Can you work these out from the model? Positions are in its coordinate system, mm. Face numbers are marked on the shaded views. A direction names the side the tool comes from. Coordinates: 2 decimals unless noted, no trailing zeros. Loops run counter-clockwise (first coordinate to the right, second up) from the corner with the lowest first, then second, coordinate; pieces in that order, holes last.
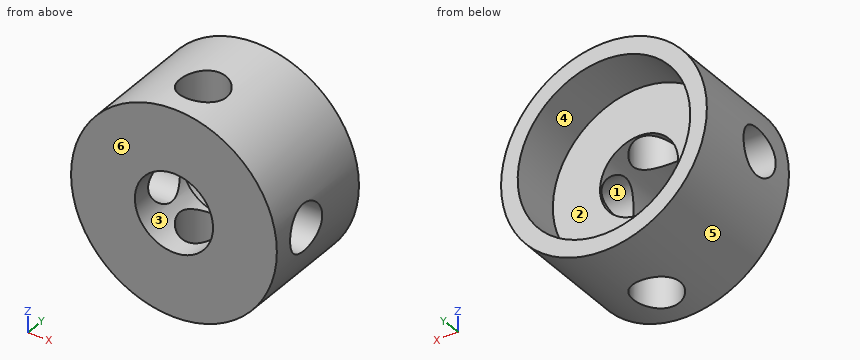
```python
from build123d import *

# Parameters (mm, degrees)
SKETCH1_R           = 7.62
SKETCH1_R_2         = 2.8956
BOSS_EXTRUDE1_DEPTH = 5.08
SKETCH2_R           = 7.62
SKETCH2_R_2         = 6.3881
BOSS_EXTRUDE2_DEPTH = 3.81
SKETCH3_R           = 1.7399
CUT_EXTRUDE1_DEPTH  = 12.7
SKETCH4_R           = 1.7399
CUT_EXTRUDE2_DEPTH  = 12.7


with BuildPart() as part:
    # Sketch1 → Boss-Extrude1 (new body)
    with BuildSketch(Plane(origin=(0, 0, 0), x_dir=(1, 0, 0), z_dir=(0, 1, 0))):
        with Locations(Location((0, 0, 0), (0, 0, 270))):
            Circle(SKETCH1_R)
        with Locations(Location((0, 0, 0), (0, 0, 270))):
            Circle(SKETCH1_R_2, mode=Mode.SUBTRACT)
    extrude(amount=BOSS_EXTRUDE1_DEPTH)

    # Sketch2 → Boss-Extrude2 (add)
    with BuildSketch(Plane(origin=(0, 5.08, 0), x_dir=(1, 0, 0), z_dir=(0, 1, 0))):
        with Locations(Location((0, 0, 0), (0, 0, 270))):
            Circle(SKETCH2_R)
        with Locations(Location((0, 0, 0), (0, 0, 90))):
            Circle(SKETCH2_R_2, mode=Mode.SUBTRACT)
    extrude(amount=BOSS_EXTRUDE2_DEPTH)

    # Sketch3 → Cut-Extrude1 (cut, symmetric)
    with BuildSketch(Plane.XY):
        with Locations((0, 3.175)):
            Circle(SKETCH3_R)
    extrude(amount=CUT_EXTRUDE1_DEPTH, both=True, mode=Mode.SUBTRACT)

    # Sketch4 → Cut-Extrude2 (cut, symmetric)
    with BuildSketch(Plane(origin=(0, 0, 0), x_dir=(0, 0, -1), z_dir=(1, 0, 0))):
        with Locations((0, 3.175)):
            Circle(SKETCH4_R)
    extrude(amount=CUT_EXTRUDE2_DEPTH, both=True, mode=Mode.SUBTRACT)


solid = part.part
```
(1) I'm going to push flat-ended pins straight in: pin 1 (4.5 mm diameter, centred on y = 3.175, z = 0, fed in from +X); pin 2 (1 mm diameter, centred on x = 4, y = 5.5, fed in from -Z). Where does each tip first touch, or does it pass through?
Check values:
pin 1: stops at x = 7.62
pin 2: stops at z = -6.77
(2) If we mould it in two halves opening along X, with no side actions, what happens to the marked faces 3, 4, 5 and 6? For each: released by +X, released by -X, zero draft, split by the parting line, or undercut.
Check values:
face 3: undercut
face 4: undercut
face 5: split by the parting line
face 6: zero draft
(3) I want a section at D-D on x = 5.5. Write out the boundary of the cut face in (y, z) (3 decimals), then the cut area to 3 significant figures.
Check values:
outline: (0, -5.274) - (8.89, -5.274) - (8.89, -3.249) - (5.08, -3.249) - (5.08, 3.249) - (8.89, 3.249) - (8.89, 5.274) - (0, 5.274) - close; hole circle Ø3.48 at (3.175, 0)
area: 59.5 mm2
(4) I want a section at A-A on x = 0. Write out the boundary of the cut face in (y, z), then the cut area to 3 significant figures.
Check values:
outline: (0, -7.62) - (1.44, -7.62) - (1.44, -2.9) - (0, -2.9) - close; (0, 2.9) - (1.44, 2.9) - (1.44, 7.62) - (0, 7.62) - close; (4.91, -7.62) - (8.89, -7.62) - (8.89, -6.39) - (5.08, -6.39) - (5.08, -2.9) - (4.91, -2.9) - close; (4.91, 2.9) - (5.08, 2.9) - (5.08, 6.39) - (8.89, 6.39) - (8.89, 7.62) - (4.91, 7.62) - close
area: 24.5 mm2
(5) I want a section at C-C on y = 6.5. Write out the boundary of the cut face in (x, z).
Check values:
outline: circle Ø15.24 at (0, 0); hole circle Ø12.78 at (0, 0)
(6) I want a section at B-B on z = 0. Write out the boundary of the cut face in (x, y), then the cut area to 3 significant figures.
Check values:
outline: (-7.62, 0) - (-2.9, 0) - (-2.9, 1.44) - (-7.62, 1.44) - close; (-7.62, 4.91) - (-2.9, 4.91) - (-2.9, 5.08) - (-6.39, 5.08) - (-6.39, 8.89) - (-7.62, 8.89) - close; (2.9, 0) - (7.62, 0) - (7.62, 1.44) - (2.9, 1.44) - close; (2.9, 4.91) - (7.62, 4.91) - (7.62, 8.89) - (6.39, 8.89) - (6.39, 5.08) - (2.9, 5.08) - close
area: 24.5 mm2
(7) If I drill on probe 1 along X at (y, z) = (7.5, -0.25); probe 2 along Y at (x, z) = (4.5, 3.5); probe 3 along Z at (x, y) = (2, 8.5), over which ranges is the centre line in solid material (lowest first)?
Check values:
probe 1: x = -7.62 to -6.38, 6.38 to 7.62
probe 2: y = 0 to 5.08
probe 3: z = -7.35 to -6.07, 6.07 to 7.35
(8) Which directions (+Z, -Z, +X, -X, +Y, -Y) give clear straight access to the entire face, cutting with the end or side of a thin tool? Please do the marked faces 1 and 2.
Check values:
face 1: +X, -X
face 2: +Y
